from build123d import *

# Parameters (mm, degrees)
SKETCH1_R            = 1.9
BOSS_EXTRUDE1_DEPTH  = 2
M4_CLEARANCE_HOLE1_D = 4.5


with BuildPart() as part:
    # Sketch1 → Boss-Extrude1 (new body)
    with BuildSketch(Plane.XY):
        with BuildLine():
            Line((-7.5, 4.5), (7.5, 4.5))
            ThreePointArc((7.5, 4.5), (12, 0), (7.5, -4.5))
            Line((7.5, -4.5), (-7.5, -4.5))
            ThreePointArc((-7.5, -4.5), (-12, 0), (-7.5, 4.5))
        make_face()
        Circle(SKETCH1_R, mode=Mode.SUBTRACT)
    extrude(amount=BOSS_EXTRUDE1_DEPTH)

    # M4 Clearance Hole1 (through all)
    with Locations(Plane.XY.offset(2)):
        with Locations((-7.5, 0), (7.5, 0)):
            Hole(M4_CLEARANCE_HOLE1_D / 2)


solid = part.part
CAD build for the part. Positions are in the model's coordinates, mm. Round coordinates to 2 decimals unless told otherwise and drop trailing zeros. Loops run counter-clockwise (first coordinate to the right, second up) from the corner with the lowest first, then second, coordinate; pieces in that order, holes last.
(1) Two-plate mould, pull along Y, no slides. Class faces 1 (the cylindrical face through (-1.9, 0.08, 0.99)), 2 (the cylindrical face through (12, 0, 1)), 3 (the flat face through (0.2, 2.1, 2)), 4 (the cylindrical face through (-5.252, 0.099, 0.986)): +Y half, -Y half, draft (parallel to the pull), parting line (faces both ways), or undercut.
(2) Wall check: line 1 along X through (y, z) = (2, 0.4); line 2 along Y through (x, z) = (-7.5, 1.4); line 3 along X through (y, z) = (1.5, 0.7). Give the ranges that are in metal, low to high.
(3) Cut at C-C (z = 1.5). Give the cut face in (x, y), plus the area to 3 significant figures.
(4) Cut at A-A (x = 0). Give the cut face in (y, z), plus the area to 3 significant figures.
(5) Cut at D-D (x = 7.75). Give the cut face in (y, z), plus the area to 3 significant figures.
(6) Drop flat-ended pins along their axis: pin 1 (4.5 mm diameter, centred on x = 0, y = 0, fed in from +Z); pin 2 (2.5 mm diameter, centred on x = -7.5, y = 0, fed in from +Z). Give the stop position or say it passes through.
(7) Cut at B-B (y = 0). Give the cut face in (x, z).
Findings below:
1. face 1: undercut
1. face 2: parting line
1. face 3: draft
1. face 4: undercut
2. line 1: x = -11.53 to -8.53, -6.47 to 6.47, 8.53 to 11.53
2. line 2: y = -4.5 to -2.25, 2.25 to 4.5
2. line 3: x = -11.74 to -9.18, -5.82 to -1.17, 1.17 to 5.82, 9.18 to 11.74
3. outline: (-7.5, -4.5) - (7.5, -4.5) arc R4.5 ccw to (7.5, 4.5) - (-7.5, 4.5) arc R4.5 ccw to start; hole circle Ø4.5 at (-7.5, 0); hole circle Ø3.8 at (0, 0); hole circle Ø4.5 at (7.5, 0)
3. area: 155 mm2
4. outline: (-4.5, 0) - (-1.9, 0) - (-1.9, 2) - (-4.5, 2) - close; (1.9, 0) - (4.5, 0) - (4.5, 2) - (1.9, 2) - close
4. area: 10.4 mm2
5. outline: (-4.49, 0) - (-2.24, 0) - (-2.24, 2) - (-4.49, 2) - close; (2.24, 0) - (4.49, 0) - (4.49, 2) - (2.24, 2) - close
5. area: 9.03 mm2
6. pin 1: stops at z = 2
6. pin 2: passes through
7. outline: (-12, 0) - (-9.75, 0) - (-9.75, 2) - (-12, 2) - close; (-5.25, 0) - (-1.9, 0) - (-1.9, 2) - (-5.25, 2) - close; (1.9, 0) - (5.25, 0) - (5.25, 2) - (1.9, 2) - close; (9.75, 0) - (12, 0) - (12, 2) - (9.75, 2) - close
